Work out the finished part from the listing and answer in its coordinate system (mm). Face numbers are marked on the shaded views. A direction names the side the tool comes from. Round coordinates to 2 decimals unless told otherwise and drop trailing zeros. Write each loop counter-clockwise with the first axis right and the second up, starting at its lowest first coordinate (ties: lowest second). Pieces come first, ordered by that corner, then holes. Notation, with made-up numbers: M 65.25,-23.5 L 84.25,-23.5 A23 ccw 84.25,-13.5 Z; hole C 60,29.5 d10. An arc over 180 degrees is marked long. One line per item, written item: value. Start each with the question number.
Q1. Find section C-C (x = 24.5). Write down the section's boundary in (y, z).
Q2. Find section D-D (y = 23). Write down the section's boundary in (x, z).
Q3. The mould has two halves that part along X. Classify the marked faces 1, 2, 3 and 4: released by +X, released by -X, zero draft, split by the parting line, or undercut.
Q4. Find section B-B (z = 9.75). Write down the section's boundary in (x, y), and give its area (3 significant figures).
Q5. Consider probe 1 along X at (y, z) = (19.5, 9.5); probe 2 along X at (y, z) = (51.5, 2); probe 3 along Y at (x, z) = (19, 12.75). Determine where each line is inside the solid, lowest interval first.
Q6. Given pin 1 Ø1.5 at (x, z) = (29, 5.5) entering from -Y; pin 2 Ø4.5 at (y, z) = (61.5, 10) entering from -X; pin 3 Ø4 at (x, z) = (9.5, 8.5) entering from -Y, each flat-ended and moving along its own axis, determine where each tip first touches the part or whether it passes through.
Q7. Find section A-A (y = 5.5). Write down the section's boundary in (x, z).
Q8. A tool of negligible diameter and unlimited length cuts with its end or side. For the marked faces 5, 6, 7 and 8, from which of +Z, -Z, +X, -X, +Y, -Y can it reach the whole face along a straight path? Write none if from no direction.
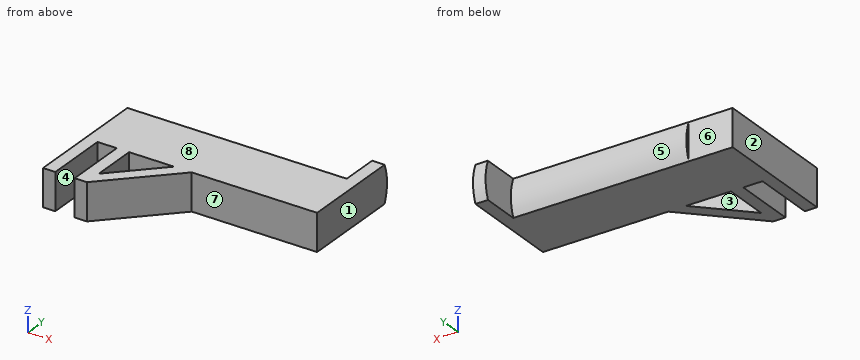
from build123d import *

# Parameters (mm, degrees)
F1_DEPTH = 14.8
F3_DEPTH = 70
F5_DEPTH = 5
F7_DEPTH = 14.8


with BuildPart() as f1:
    # F0 (on Top) → F1 (new body)
    with BuildSketch(Plane.XY):
        Polygon((0, 50), (0, 0), (4.9, 0), (4.9, 25), (12.6, 25), (12.6, 0), (17.5, 0), (17.5, 50), align=None)
    extrude(amount=F1_DEPTH)

    # F2 (on face) → F3 (join)
    with BuildSketch(Plane.YZ.offset(17.5)):
        with BuildLine():
            ThreePointArc((50, 0), (51.419365, 7.4), (50, 14.8))
            Line((50, 14.8), (25, 14.8))
            Line((25, 14.8), (25, 0))
            Line((25, 0), (50, 0))
        make_face()
    extrude(amount=F3_DEPTH)

    # F4 (on face) → F5 (join)
    with BuildSketch(Plane.YZ.offset(87.5)):
        with BuildLine():
            Line((65, 14.8), (25, 14.8))
            Line((25, 14.8), (25, 0))
            Line((25, 0), (65, 0))
            ThreePointArc((65, 0), (66.419365, 7.4), (65, 14.8))
        make_face()
    extrude(amount=F5_DEPTH)

    # F6 (on face) → F7 (join, through all)
    with BuildSketch(Plane.XY.offset(14.8)):
        Polygon((17.5, 7.071068), (17.5, 0), (42.5, 25), (35.428932, 25), align=None)
    extrude(amount=-F7_DEPTH)


solid = f1.part
The answers:
1. outline: M 7,0 L 14.07,0 L 14.07,14.8 L 7,14.8 Z; M 25,0 L 50,0 A20 ccw 50,14.8 L 25,14.8 Z
2. outline: M 0,0 L 4.9,0 L 4.9,14.8 L 0,14.8 Z; M 12.6,0 L 17.5,0 L 17.5,14.8 L 12.6,14.8 Z; M 33.43,0 L 40.5,0 L 40.5,14.8 L 33.43,14.8 Z
3. face 1: released by +X
3. face 2: released by -X
3. face 3: undercut
3. face 4: undercut
4. outline: M 0,0 L 4.9,0 L 4.9,25 L 12.6,25 L 12.6,0 L 17.5,0 L 42.5,25 L 92.5,25 L 92.5,66.28 L 87.5,66.28 L 87.5,51.28 L 17.5,51.28 L 17.5,50 L 0,50 Z; hole M 17.5,7.07 L 35.43,25 L 17.5,25 Z
4. area: 2,880 mm2
5. probe 1: 0 to 4.9, 12.6 to 17.5, 29.93 to 37
5. probe 2: 87.5 to 92.5
5. probe 3: 1.5 to 8.57, 25 to 50.69
6. pin 1: y = 10.75
6. pin 2: x = 87.5
6. pin 3: y = 25
7. outline: M 0,0 L 4.9,0 L 4.9,14.8 L 0,14.8 Z; M 12.6,0 L 23,0 L 23,14.8 L 12.6,14.8 Z
8. face 5: -X, +Y
8. face 6: +Z, -Z, -X, +Y
8. face 7: +Z, -Z, +X, -Y
8. face 8: +Z, +X, -X, +Y, -Y
